from build123d import *

# Parameters (mm, degrees)
BOSS_EXTRUDE1_DEPTH = 70
SKETCH2_R           = 1.5
CUT_EXTRUDE1_DEPTH  = 17.390666387


with BuildPart() as part:
    # Sketch1 → Boss-Extrude1 (new body)
    with BuildSketch(Plane.YZ):
        with BuildLine():
            ThreePointArc((17.390666387, -60), (9.790666387, -67.6), (17.390666387, -75.2))
            Line((17.390666387, -75.2), (17.390666387, -85.2))
            Line((17.390666387, -85.2), (0, -85.2))
            Line((0, -85.2), (0, 0))
            Line((0, 0), (17.390666387, 0))
            Line((17.390666387, 0), (17.390666387, -10))
            ThreePointArc((17.390666387, -10), (9.790666387, -17.6), (17.390666387, -25.2))
            Line((17.390666387, -25.2), (17.390666387, -60))
        make_face()
    extrude(amount=BOSS_EXTRUDE1_DEPTH)

    # Sketch2 → Cut-Extrude1 (cut)
    with BuildSketch(Plane(origin=(0, 17.390666387, 0), x_dir=(-1, 0, 0), z_dir=(0, 1, 0))):
        with Locations(Location((-52.5, -5, 0), (0, 0, 90))):
            Circle(SKETCH2_R)
        with Locations(Location((-17.5, -5, 0), (0, 0, 90))):
            Circle(SKETCH2_R)
        with Locations(Location((-52.5, -80.2, 0), (0, 0, 90))):
            Circle(SKETCH2_R)
        with Locations(Location((-17.5, -80.2, 0), (0, 0, 90))):
            Circle(SKETCH2_R)
        with Locations(Location((-35, -30.2, 0), (0, 0, 90))):
            Circle(SKETCH2_R)
        with Locations(Location((-35, -55, 0), (0, 0, 90))):
            Circle(SKETCH2_R)
    extrude(amount=-CUT_EXTRUDE1_DEPTH, mode=Mode.SUBTRACT)


solid = part.part
Geometry check sheet. Reference: the model listing, model coordinates, mm. Give positions to 0.01 mm unless a question says otherwise; leave off trailing zeros. Order: outer loops, then holes, each group sorted by start corner. A loop starts at its lowest first (then second) coordinate and runs counter-clockwise, first axis right, second up.
1. Draft check along Z on faces 1 (the face through (51.17, 8.82, -79.51)), 2 (the face through (35, 9, 0)), 3 (the face through (35, 17.391, -42)). Enter one of: pulls with the +Z half, pulls with the -Z half, needs draft (parallel to the pull), parting line crosses it, or undercut.
Completed:
face 1: undercut
face 2: pulls with the +Z half
face 3: needs draft
2. Scan lines: line 1 (X direction, y = 5, z = -80.2); line 2 (X direction, y = 5.25, z = -55); line 3 (X direction, y = 5.5, z = -79). Record each from-to range of solid material in increasing order.
Completed:
line 1: x = 0 to 16, 19 to 51, 54 to 70
line 2: x = 0 to 33.5, 36.5 to 70
line 3: x = 0 to 16.6, 18.4 to 51.6, 53.4 to 70
3. Depth check by flat-ended pin: pin 1 (2.5 mm diameter, centred on x = 52.5, z = -80.2, fed in from +Y). Enter the tip coordinate at first touch or a pass-through.
Completed:
pin 1: passes through
4. Sectioned sample at B-B (z = -30.2). Record the boundary of the cut face in (x, y), then the cut area to 3 significant figures.
Completed:
outline: (0, 0) - (33.5, 0) - (33.5, 17.39) - (0, 17.39) - close; (36.5, 0) - (70, 0) - (70, 17.39) - (36.5, 17.39) - close
area: 1,170 mm2
5. Sectioned sample at A-A (z = -80.2). Record the boundary of the cut face in (x, y).
Completed:
outline: (0, 0) - (16, 0) - (16, 17.39) - (0, 17.39) - close; (19, 0) - (51, 0) - (51, 17.39) - (19, 17.39) - close; (54, 0) - (70, 0) - (70, 17.39) - (54, 17.39) - close
6. Sectioned sample at D-D (y = 14.25). State how many separate pieces and enclosed holes the cut face has, then the cut area to 3 significant figures.
Completed:
separate pieces: 3
enclosed holes: 6
area: 3,980 mm2
7. Sectioned sample at C-C (x = 52.5). Record the boundary of the cut face in (y, z).
Completed:
outline: (0, -85.2) - (17.39, -85.2) - (17.39, -81.7) - (0, -81.7) - close; (0, -78.7) - (17.39, -78.7) - (17.39, -75.2) arc R7.6 cw to (17.39, -60) - (17.39, -25.2) arc R7.6 cw to (17.39, -10) - (17.39, -6.5) - (0, -6.5) - close; (0, -3.5) - (17.39, -3.5) - (17.39, 0) - (0, 0) - close
